Geometry check sheet. Reference: drawing and pictorial views, mm from the part's lowest x, y, z. A direction names the side the tool comes from. Give positions to 0.01 mm unless a question says otherwise; leave off trailing zeros. Loops run counter-clockwise (first coordinate to the right, second up) from the corner with the lowest first, then second, coordinate; pieces in that order, holes last. Notation, with made-up numbers: M -7.5,4 L 25.5,4 A14 ccw 25.5,31 Z; hole C 27.25,-31.75 d11. An arc over 180 degrees is marked long. Use CSV: the item, a comma, the result in double quotes.
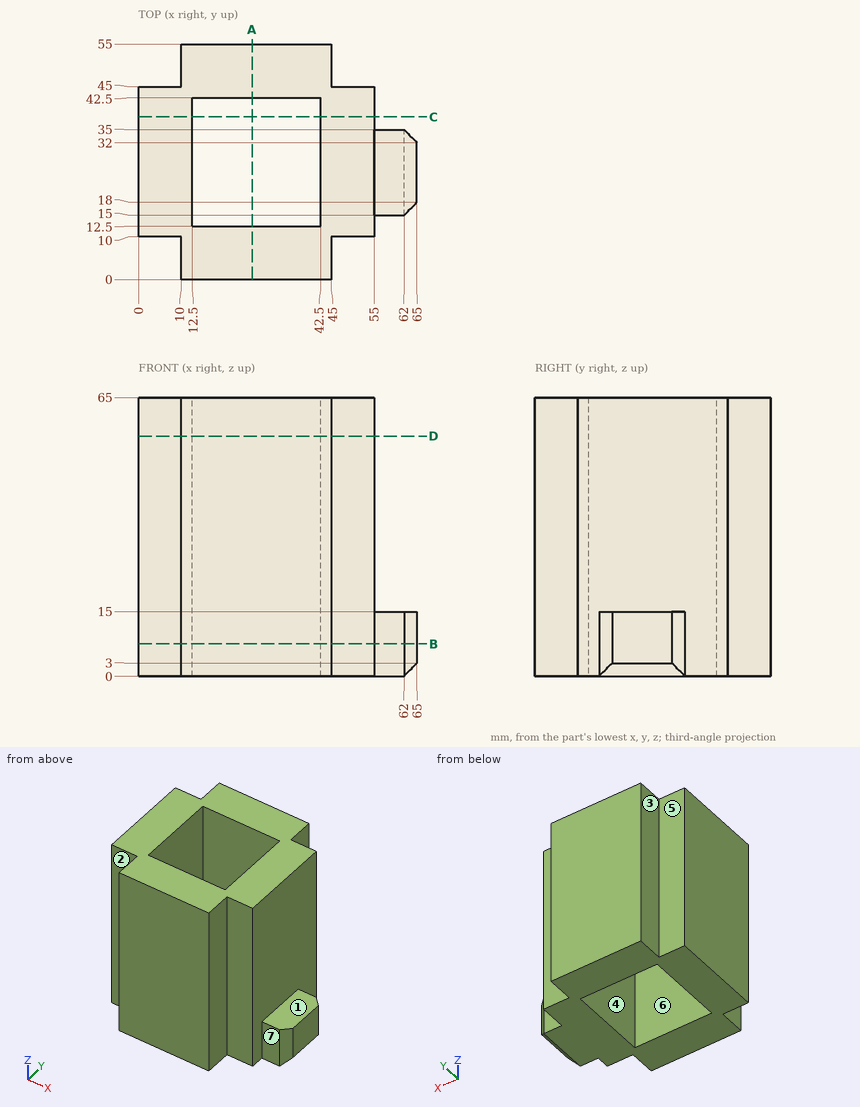
(1) Scan lines: L1, parallel to X at y = 17.5, z = 40; L2, parallel to X at y = 29, z = 7. Record each from-to range of solid material in increasing order. Write a range as from..to.
Calculated:
L1,"x = 0..12.5, 42.5..55"
L2,"x = 0..12.5, 42.5..65"
(2) Depth check by flat-ended pin: pin 1 Ø1.5 at (y, z) = (34.5, 32.5) entering from +X; pin 2 Ø1.5 at (x, z) = (6.5, 20) entering from +Y; pin 3 Ø3 at (x, z) = (4, 28.5) entering from -Y. Enter the tip coordinate at first touch or a pass-through.
Calculated:
pin 1,"stops at x = 55"
pin 2,"stops at y = 45"
pin 3,"stops at y = 10"
(3) Mould release check, pull along Y, two halves, no side actions. Record for the marked faces 4, 5, 6 and 7: released by +Y, released by -Y, zero draft, split by the parting line, or undercut.
Calculated:
face 4,"undercut"
face 5,"released by +Y"
face 6,"undercut"
face 7,"released by -Y"
(4) Section check D-D on z = 56. Record the cut outline in (x, y), plus the area to 4 significant figures.
Calculated:
outline,"M 0,10 L 10,10 L 10,0 L 45,0 L 45,10 L 55,10 L 55,45 L 45,45 L 45,55 L 10,55 L 10,45 L 0,45 Z; hole M 12.5,12.5 L 42.5,12.5 L 42.5,42.5 L 12.5,42.5 Z"
area,"1,725 mm²"
(5) Section check B-B on z = 7.5. Record the cut outline in (x, y).
Calculated:
outline,"M 0,10 L 10,10 L 10,0 L 45,0 L 45,10 L 55,10 L 55,15 L 62,15 L 65,18 L 65,32 L 62,35 L 55,35 L 55,45 L 45,45 L 45,55 L 10,55 L 10,45 L 0,45 Z; hole M 12.5,12.5 L 42.5,12.5 L 42.5,42.5 L 12.5,42.5 Z"
(6) Tool access check on the marked faces 1, 2 and 3. Record the directions out of +Z, -Z, +X, -X, +Y, -Y that give a thin tool (end or side, any length) a straight path to the whole face; none if there is none.
Calculated:
face 1,"+Z, +X, +Y, -Y"
face 2,"+Z, -Z, -X, -Y"
face 3,"+Z, -Z, -X, +Y"
(7) Section check A-A on x = 26.5. Record the cut outline in (y, z), plus the area to 4 significant figures.
Calculated:
outline,"M 0,0 L 12.5,0 L 12.5,65 L 0,65 Z; M 42.5,0 L 55,0 L 55,65 L 42.5,65 Z"
area,"1,625 mm²"
